```python
from build123d import *

# Parameters (mm, degrees)
F0_R     = 50.8
F0_R_2   = 44.45
F0_R_3   = 11.176
F1_DEPTH = 12.7
F2_R     = 6.35
F2_R_2   = 11.176
F3_DEPTH = 12.701
F2_R_3   = 50.8
F2_R_4   = 44.45
F4_DEPTH = 12.7


# Not quite as in the source:
# - a feature names something its author has since deleted; it is built from what else it names


with BuildPart() as f1:
    # F0 (on Front) → F1 (new body)
    with BuildSketch(Plane.XZ):
        Circle(F0_R)
        Circle(F0_R_2, mode=Mode.SUBTRACT)
        Circle(F0_R_2)
        Circle(F0_R_3, mode=Mode.SUBTRACT)
        Circle(F0_R_3)
    extrude(amount=F1_DEPTH)

    # F2 (on face) → F3 (cut, through all)
    with BuildSketch(Plane.XZ.offset(12.7)):
        with Locations((0, 28.575)):
            Circle(F2_R)
        with Locations((-24.7466759131, -14.2875)):
            Circle(F2_R)
        Circle(F2_R_2)
        with Locations((24.7466759131, -14.2875)):
            Circle(F2_R)
    extrude(amount=-F3_DEPTH, mode=Mode.SUBTRACT)

    # F2 (on face) → F4 (join)
    with BuildSketch(Plane.XZ.offset(12.7)):
        Circle(F2_R_3)
        Circle(F2_R_4, mode=Mode.SUBTRACT)
    extrude(amount=F4_DEPTH)


solid = f1.part
```
The model under review builds one solid part; all positions refer to its coordinate system, in mm. A direction names the side the tool comes from. Coordinates: 2 decimals unless noted, no trailing zeros. Write each loop counter-clockwise with the first axis right and the second up, starting at its lowest first coordinate (ties: lowest second). Pieces come first, ordered by that corner, then holes. Notation, with made-up numbers: (-24.5, -32) -> (1.5, -32) arc R22 cw to (1.5, -9) -> close; hole circle Ø7 at (72.5, -7.5). An arc over 180 degrees is marked (long way). One line per item, written item: value. Start each with the question number.
Q1. For faces 4 (the face through (42.397, -18.961, 13.352)), 5 (the face through (-1.377, -6.439, 22.376)), list the 3-axis set-ups (+Z, -Z, +X, -X, +Y, -Y) from which the entire face can be reached by the end or side of a thin tool; tool diameter is ignored.
Q2. Add section A-A, the plane x = 0. Give the boundary of the cut face in (y, z) (3 decimals).
Q3. Clearance check with flat-ended pins moving along their axes: P1, Ø2, axis at y = -10.5, z = -19.5, coming from the +X side; P2, Ø8, axis at x = -30.5, z = -3, coming from the -Y side; P3, Ø6, axis at x = -29, y = -10.5, coming from the -Z side; P4, Ø11.5, axis at x = -24.75, z = -14.29, coming from the -Y side. State where each tip first meets the part, or that it passes through.
Q4. Add section D-D, the plane y = -15.75. Give the boundary of the cut face in (x, z), then the cut area to 3 significant figures.
Q5. Add section C-C, the plane x = 24.5. Give the boundary of the cut face in (y, z).
Q6. The part is to be moulded in two halves that separate along Z. For faces 1 (the face through (9, -12.7, -9)), 2 (the face through (-11.012, -12.522, -49.592)), 3 (the face through (-12, 0, 1)), say which applies: +Z half, -Z half, draft (parallel to the pull), parting line (faces both ways), or undercut.
Q7. Add section B-B, the plane z = 0. Give the boundary of the cut face in (x, y).
Q8. To check wall thickness, follow probe 1 along Z at (x, y) = (0, -7) (3 decimals); probe 2 along Z at (x, y) = (0, -17.5); probe 3 along X at (y, z) = (-3, -10). State the ranges of each line that lie inside material, in increasing order.
Response:
1. face 4: -Y
1. face 5: +Y, -Y
2. outline: (-25.4, -50.8) -> (0, -50.8) -> (0, -11.176) -> (-12.7, -11.176) -> (-12.7, -44.45) -> (-25.4, -44.45) -> close; (-25.4, 44.45) -> (-12.7, 44.45) -> (-12.7, 34.925) -> (0, 34.925) -> (0, 50.8) -> (-25.4, 50.8) -> close; (-12.7, 11.176) -> (0, 11.176) -> (0, 22.225) -> (-12.7, 22.225) -> close
3. P1: x = 47.31
3. P2: y = -12.7
3. P3: z = -43.64
3. P4: through
4. outline: circle Ø101.6 at (0, 0); hole circle Ø88.9 at (0, 0)
4. area: 1,900 mm²
5. outline: (-25.4, -44.5) -> (0, -44.5) -> (0, -20.63) -> (-12.7, -20.63) -> (-12.7, -37.09) -> (-25.4, -37.09) -> close; (-25.4, 37.09) -> (-12.7, 37.09) -> (-12.7, -7.94) -> (0, -7.94) -> (0, 44.5) -> (-25.4, 44.5) -> close
6. face 1: undercut
6. face 2: parting line
6. face 3: draft
7. outline: (-50.8, -25.4) -> (-44.45, -25.4) -> (-44.45, -12.7) -> (-11.18, -12.7) -> (-11.18, 0) -> (-50.8, 0) -> close; (11.18, -12.7) -> (44.45, -12.7) -> (44.45, -25.4) -> (50.8, -25.4) -> (50.8, 0) -> (11.18, 0) -> close
8. probe 1: -50.8 to -11.176, 11.176 to 22.225, 34.925 to 50.8
8. probe 2: -50.8 to -44.45, 44.45 to 50.8
8. probe 3: -49.81 to -29.43, -20.06 to -4.99, 4.99 to 20.06, 29.43 to 49.81
